```python
from build123d import *

# Parameters (mm, degrees)
SKETCH2_W           = 86
SKETCH2_H           = 86
SKETCH2_W_2         = 42
SKETCH2_H_2         = 42
BOSS_EXTRUDE1_DEPTH = 3
SKETCH3_R           = 3.25
CUT_EXTRUDE1_DEPTH  = 3
SKETCH7_R           = 2.25
CUT_EXTRUDE2_DEPTH  = 3
FILLET1_R           = 5
FILLET2_R           = 5
FILLET3_R           = 5
FILLET4_R           = 5


with BuildPart() as part:
    # Sketch2 → Boss-Extrude1 (new body)
    with BuildSketch(Plane(origin=(0, 0, 0), x_dir=(1, 0, 0), z_dir=(0, 1, 0))):
        with Locations((1.854851242, 27.411515707)):
            Rectangle(SKETCH2_W, SKETCH2_H)
        with Locations((1.854851242, 27.411515707)):
            Rectangle(SKETCH2_W_2, SKETCH2_H_2, mode=Mode.SUBTRACT)
    extrude(amount=BOSS_EXTRUDE1_DEPTH)

    # Sketch3 → Cut-Extrude1 (cut)
    with BuildSketch(Plane(origin=(0, 3, 0), x_dir=(1, 0, 0), z_dir=(0, 1, 0))):
        with Locations((34.854851242, -5.588484293)):
            Circle(SKETCH3_R)
        with Locations((-31.145148758, -5.588484293)):
            Circle(SKETCH3_R)
        with Locations((-31.145148758, 60.411515707)):
            Circle(SKETCH3_R)
        with Locations((34.854851242, 60.411515707)):
            Circle(SKETCH3_R)
    extrude(amount=-CUT_EXTRUDE1_DEPTH, mode=Mode.SUBTRACT)

    # Sketch7 → Cut-Extrude2 (cut)
    with BuildSketch(Plane(origin=(0, 3, 0), x_dir=(1, 0, 0), z_dir=(0, 1, 0))):
        with Locations((26.390385148, 2.875981801)):
            Circle(SKETCH7_R)
        with Locations((-22.680682664, 2.875981801)):
            Circle(SKETCH7_R)
        with Locations((-22.680682664, 51.947049613)):
            Circle(SKETCH7_R)
        with Locations((26.390385148, 51.947049613)):
            Circle(SKETCH7_R)
    extrude(amount=-CUT_EXTRUDE2_DEPTH, mode=Mode.SUBTRACT)

    # Fillet1
    fillet1_edges = [part.edges().sort_by_distance(p)[0] for p in [
        (-41.145148758, 1.5, -70.411515707),
    ]]
    fillet(fillet1_edges, radius=FILLET1_R)

    # Fillet2
    fillet2_edges = [part.edges().sort_by_distance(p)[0] for p in [
        (44.854851242, 1.5, 15.588484293),
    ]]
    fillet(fillet2_edges, radius=FILLET2_R)

    # Fillet3
    fillet3_edges = [part.edges().sort_by_distance(p)[0] for p in [
        (-41.145148758, 1.5, 15.588484293),
    ]]
    fillet(fillet3_edges, radius=FILLET3_R)

    # Fillet4
    fillet4_edges = [part.edges().sort_by_distance(p)[0] for p in [
        (44.854851242, 1.5, -70.411515707),
    ]]
    fillet(fillet4_edges, radius=FILLET4_R)


solid = part.part
```
Can you work these out from the model? Positions are in its coordinate system, mm. A direction names the side the tool comes from. Round coordinates to 2 decimals unless told otherwise and drop trailing zeros. Loops run counter-clockwise (first coordinate to the right, second up) from the corner with the lowest first, then second, coordinate; pieces in that order, holes last. Notation, with made-up numbers: (-37.75, 76) -> (-20.75, 76) arc R10 cw to (-20.75, 90) -> close; hole circle Ø6 at (73, 31). An arc over 180 degrees is marked (long way). One line per item, written item: value. Start each with the question number.
1. If we section it at B-B, the plane z = -19: Write out the boundary of the cut face in (x, y).
2. If we section it at C-C, the plane x = 37: Write out the boundary of the cut face in (y, z).
3. If we section it at A-A, the plane x = -17.5: Write out the boundary of the cut face in (y, z).
4. If we mould it in two halves opening along Z, with no side actions, what happens to faces 1 (the flat face through (1, 1, -70.412)), 2 (the flat face through (2, 1, -48.412)), 3 (the flat face through (44.855, 1, -27))? For each: pulls with the +Z half, pulls with the -Z half, needs draft (parallel to the pull), parting line crosses it, or undercut.
5. If I drill on probe 1 along X at (y, z) = (2.35, -13.5); probe 2 along X at (y, z) = (2.6, 6); probe 3 along Z at (x, y) = (-34, 1.6), over which ranges is the centre line in solid material (lowest first)?
6. For faces 4 (the flat face through (-41.145, 1, -27)), 5 (the flat face through (-19.145, 1, -27)), which set-ups out of +Z, -Z, +X, -X, +Y, -Y let a thin tool reach every point of the face, with its end or its side?
7. For pin 1 (5 mm diameter, centred on x = -31.15, z = -60.41, fed in from +Y), with a flat end and sliding along its axis, tell me the tip position at first contact or that it passes through.
8. If we section it at D-D, the plane y = 0.45: Give the number of separate pieces and of enclosed holes in the cut face, then the cut area to 3 significant figures.
Calculated:
1. outline: (-41.15, 0) -> (-19.15, 0) -> (-19.15, 3) -> (-41.15, 3) -> close; (22.85, 0) -> (44.85, 0) -> (44.85, 3) -> (22.85, 3) -> close
2. outline: (0, -70.41) -> (3, -70.41) -> (3, -62.85) -> (0, -62.85) -> close; (0, -57.97) -> (3, -57.97) -> (3, 3.15) -> (0, 3.15) -> close; (0, 8.03) -> (3, 8.03) -> (3, 15.59) -> (0, 15.59) -> close
3. outline: (0, -70.41) -> (3, -70.41) -> (3, -48.41) -> (0, -48.41) -> close; (0, -6.41) -> (3, -6.41) -> (3, 15.59) -> (0, 15.59) -> close
4. face 1: pulls with the -Z half
4. face 2: undercut
4. face 3: needs draft
5. probe 1: x = -41.15 to -19.15, 22.85 to 44.85
5. probe 2: x = -41.15 to -34.37, -27.92 to 31.63, 38.08 to 44.85
5. probe 3: z = -70.41 to -61.96, -58.86 to 4.04, 7.14 to 15.59
6. face 4: +Z, -Z, -X, +Y, -Y
6. face 5: +Y, -Y
7. pin 1: passes through
8. separate pieces: 1
8. enclosed holes: 9
8. area: 5,410 mm²
